from build123d import *

# Parameters (mm, degrees)
SKETCH2_W           = 72.654814815
SKETCH2_H           = 58.693333333
SKETCH2_W_2         = 69.44
SKETCH2_H_2         = 54.5
BOSS_EXTRUDE1_DEPTH = 5
SKETCH3_W           = 5
SKETCH3_H           = 10
CUT_EXTRUDE1_DEPTH  = 10
CUT_EXTRUDE4_DEPTH  = 10


with BuildPart() as part:
    # Sketch2 → Boss-Extrude1 (new body)
    with BuildSketch(Plane.XY):
        with Locations((-0.551111111, -3.352592593)):
            Rectangle(SKETCH2_W, SKETCH2_H)
        with Locations((-0.321481481, -3.092962963)):
            Rectangle(SKETCH2_W_2, SKETCH2_H_2, mode=Mode.SUBTRACT)
    extrude(amount=BOSS_EXTRUDE1_DEPTH)

    # Sketch3 → Cut-Extrude1 (cut)
    with BuildSketch(Plane(origin=(35.776296296, 0, 0), x_dir=(0, 0, -1), z_dir=(1, 0, 0))):
        with Locations((-2.5, 14.994074074)):
            Rectangle(SKETCH3_W, SKETCH3_H)
    extrude(amount=-CUT_EXTRUDE1_DEPTH, mode=Mode.SUBTRACT)

    # Sketch4 → Cut-Extrude4 (cut)
    with BuildSketch(Plane(origin=(35.776296296, 0, 0), x_dir=(0, 0, -1), z_dir=(1, 0, 0))):
        Polygon((-5, -10.699259259), (-5, -22.699259259), (0, -22.699259259), (0, -10.699259259), (0, 9.994074074), (-5, 9.994074074), align=None)
    extrude(amount=-CUT_EXTRUDE4_DEPTH, mode=Mode.SUBTRACT)


solid = part.part
CAD build for the part. Positions are in the model's coordinates, mm. A direction names the side the tool comes from. Round coordinates to 2 decimals unless told otherwise and drop trailing zeros. Order: outer loops, then holes, each group sorted by start corner. A loop starts at its lowest first (then second) coordinate and runs counter-clockwise, first axis right, second up. Notation, with made-up numbers: (5.25, 86.5) -> (59.25, 86.5) arc R18 ccw to (59.25, 92.5) -> close; hole circle Ø3 at (57, -17.5). An arc over 180 degrees is marked (long way). Write item = value, one per line. Start each with the question number.
(1) Probe line 1 (Y direction, x = -15, z = 3.45); line 2 (X direction, y = -23.5, z = 2.55); line 3 (X direction, y = 9, z = 2.5). List the from-to ranges inside material, lowest first. Write a range as [from, to].
(2) Cut at A-A, the plane x = 23.5. List the corners of the cut face in (y, z), then the cut area to 3 significant figures.
(3) Which spindle directions (+Z, -Z, +X, -X, +Y, -Y) get a long thin tool onto all of the face, cutting with end or side? Do faces 1 (the flat face through (-36, -3, 0)), 2 (the flat face through (34.399, 22, 2)). Say none if no direction does.
(4) Pull direction X, two halves, no side cores. Call faces 3 (the flat face through (-1, 25.994, 2)), 4 (the flat face through (34.399, -27, 2)), 5 (the flat face through (-36.879, -4, 2)), 6 (the flat face through (-1, -30.343, 2)): released by +X, released by -X, zero draft, split by the parting line, or undercut.
(5) Cut at C-C, the plane y = -12.5. List the corners of the cut face in (x, z).
(6) Cut at B-B, the plane z = 1.7. List the corners of the cut face in (x, y), then the cut area to 3 significant figures.
Model answer:
q1.line_1 = [-32.7, -30.34], [24.16, 25.99]
q1.line_2 = [-36.88, -35.04], [34.4, 35.78]
q1.line_3 = [-36.88, -35.04]
q2.outline = (-32.7, 0) -> (-30.34, 0) -> (-30.34, 5) -> (-32.7, 5) -> close; (24.16, 0) -> (25.99, 0) -> (25.99, 5) -> (24.16, 5) -> close
q2.area = 21.0 mm2
q3.face_1 = -Z, +X, -X, +Y, -Y
q3.face_2 = +Z, -Z
q4.face_3 = zero draft
q4.face_4 = undercut
q4.face_5 = released by -X
q4.face_6 = undercut
q5.outline = (-36.88, 0) -> (-35.04, 0) -> (-35.04, 5) -> (-36.88, 5) -> close
q6.outline = (-36.88, -32.7) -> (35.78, -32.7) -> (35.78, -22.7) -> (34.4, -22.7) -> (34.4, -30.34) -> (-35.04, -30.34) -> (-35.04, 24.16) -> (34.4, 24.16) -> (34.4, 19.99) -> (35.78, 19.99) -> (35.78, 25.99) -> (-36.88, 25.99) -> close
q6.area = 421 mm2
